For this review, take the finished solid that the model builds, in its own axes (mm). Face numbers are marked on the shaded views. Round coordinates to 2 decimals unless told otherwise and drop trailing zeros. Order: outer loops, then holes, each group sorted by start corner. A loop starts at its lowest first (then second) coordinate and runs counter-clockwise, first axis right, second up. Notation, with made-up numbers: M 25.25,51.5 L 65.25,51.5 A15 cw 65.25,79.5 Z; hole C 47.25,42 d7. An arc over 180 degrees is marked long. Write item = value, one per line. Start each with the question number.
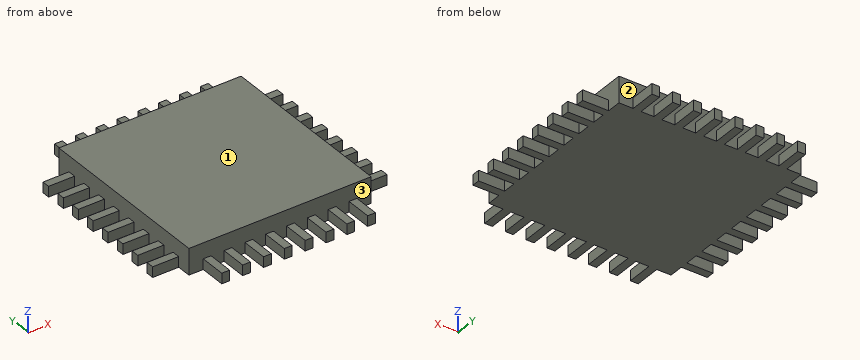
from build123d import *

# Parameters (mm, degrees)
F0_W     = 7
F0_H     = 7
F1_DEPTH = 1
F2_W     = 1
F2_H     = 0.3
F3_DEPTH = 0.4
F5_COUNT = 4
F5_ANGLE = 270


with BuildPart() as f1:
    # F0 (on Top) → F1 (new body)
    with BuildSketch(Plane.XY):
        Rectangle(F0_W, F0_H)
    extrude(amount=F1_DEPTH)

    # F2 (on Top) → F3 (join)
    with BuildSketch(Plane.XY):
        with Locations((-4, 2.8)):
            Rectangle(F2_W, F2_H)
        with Locations((-4, 2)):
            Rectangle(F2_W, F2_H)
        with Locations((-4, 1.2)):
            Rectangle(F2_W, F2_H)
        with Locations((-4, -1.2)):
            Rectangle(F2_W, F2_H)
        with Locations((-4, 0.4)):
            Rectangle(F2_W, F2_H)
        with Locations((-4, -0.4)):
            Rectangle(F2_W, F2_H)
        with Locations((-4, -2)):
            Rectangle(F2_W, F2_H)
        with Locations((-4, -2.8)):
            Rectangle(F2_W, F2_H)
    extrude(amount=F3_DEPTH)

    # F5: F1 ×4 about axis
    f5_axis = Axis((0, 0, 4.798143), (0, 0, 1))


with BuildPart() as f1_1:
    add(f1.part)
    for i in range(1, F5_COUNT):
        add(f1.part.rotate(f5_axis, i * F5_ANGLE / (F5_COUNT - 1)))


solid = f1_1.part
(1) Draft analysis for pull direction X (two halves, no side actions). For the marked faces 1, 2 and 3, state which applies: released by +X, released by -X, zero draft, split by the parting line, or undercut.
(2) For line 1 along Y through (x, z) = (-2.5, 0.75); line 2 along Z through (x, y) = (2, 4.25), list the stretches that pass through material, from the lowest coordinate up.
(3) We need section B-B, the plane x = 3.25. Write out the cut boundary in (y, z).
(4) We need section A-A, the plane y = 4.25. State how many separate pieces and enclosed holes the cut face has, then the cut area to 3 significant figures.
(5) Insertion check: pin 1 (1.5 mm diameter, centred on x = 0, y = 0, fed in from -Z). The pin has a flat end and moves straight along its axis. Give the tip position at first contact, or say it passes through.
Values:
q1.face_1 = zero draft
q1.face_2 = undercut
q1.face_3 = undercut
q2.line_1 = -3.5 to 3.5
q2.line_2 = 0 to 0.4
q3.outline = M -3.5,0 L 3.5,0 L 3.5,1 L -3.5,1 Z
q4.separate_pieces = 8
q4.enclosed_holes = 0
q4.area = 0.960 mm²
q5.pin_1 = 0
